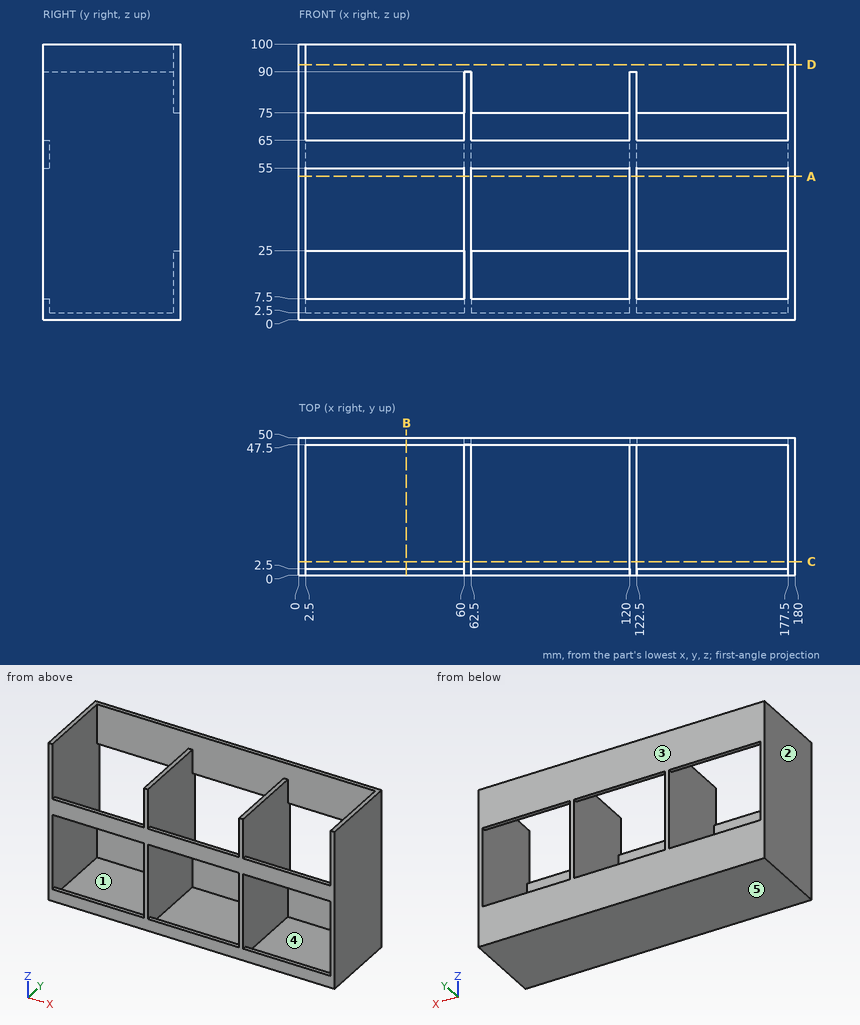
Could you check a few things on this drawing? It's one solid part, dimensions in mm from its lowest x, y, z. A direction names the side the tool comes from. Give positions to 0.01 mm unless a question says otherwise; leave off trailing zeros. Loops run counter-clockwise (first coordinate to the right, second up) from the corner with the lowest first, then second, coordinate; pieces in that order, holes last. Notation, with made-up numbers: M 33.5,10 L 48.5,10 A20 cw 48.5,35 Z; hole C 13,72.5 d9. An arc over 180 degrees is marked long. Answer as a JSON object with one key per item and string values.
Q1. Suppose I cut it at B-B, the plane x = 39. List the corners of the cut face in (y, z) for me.
Values found:
{"outline": "M 0,0 L 50,0 L 50,25 L 47.5,25 L 47.5,2.5 L 2.5,2.5 L 2.5,7.5 L 0,7.5 Z; M 0,55 L 2.5,55 L 2.5,65 L 0,65 Z; M 47.5,75 L 50,75 L 50,100 L 47.5,100 Z"}
Q2. Suppose I cut it at D-D, the plane z = 92.5. List the corners of the cut face in (x, y) for me.
Values found:
{"outline": "M 0,0 L 2.5,0 L 2.5,47.5 L 177.5,47.5 L 177.5,0 L 180,0 L 180,50 L 0,50 Z"}
Q3. For P1, Ø8, axis at y = 22.5, z = 55.5, coming from the -X side; P2, Ø22.5, axis at x = 96.5, y = 31.5, coming from the +Z side; P3, Ø3, axis at x = 85.5, y = 1.5, coming from the +Z side; P4, Ø11, axis at x = 82.5, z = 59.5, coming from the +Y side, each with a flat end and sliding along its axis, tell me the tip position at first contact or that it passes through.
Values found:
{"P1": "stops at x = 0", "P2": "stops at z = 2.5", "P3": "stops at z = 65", "P4": "stops at y = 2.5"}
Q4. If we mould it in two halves opening along X, with no side actions, what happens to the marked faces 1, 2 and 3? For each: pulls with the +X half, pulls with the -X half, needs draft (parallel to the pull), parting line crosses it, or undercut.
Values found:
{"face 1": "undercut", "face 2": "pulls with the -X half", "face 3": "needs draft"}
Q5. Suppose I cut it at A-A, the plane z = 52. List the corners of the cut face in (x, y) for me, plus the area to 3 significant figures.
Values found:
{"outline": "M 0,0 L 2.5,0 L 2.5,50 L 0,50 Z; M 60,0 L 62.5,0 L 62.5,50 L 60,50 Z; M 120,0 L 122.5,0 L 122.5,50 L 120,50 Z; M 177.5,0 L 180,0 L 180,50 L 177.5,50 Z", "area": "500 mm²"}
Q6. For the marked faces 4 and 5, which set-ups out of +Z, -Z, +X, -X, +Y, -Y let a thin tool reach every point of the face, with its end or its side?
Values found:
{"face 4": "+Z", "face 5": "-Z, +X, -X, +Y, -Y"}
Q7. If I drill on probe 1 along X at (y, z) = (11.5, 78.5); probe 2 along X at (y, z) = (5.5, 91); probe 3 along Z at (x, y) = (171, 41.5), over which ranges is the centre line in solid material (lowest first)? Write a range as [from, to].
Values found:
{"probe 1": "x = [0, 2.5], [60, 62.5], [120, 122.5], [177.5, 180]", "probe 2": "x = [0, 2.5], [177.5, 180]", "probe 3": "z = [0, 2.5]"}
Q8. Suppose I cut it at C-C, the plane y = 5. List the corners of the cut face in (x, z) for me, plus the area to 4 significant figures.
Values found:
{"outline": "M 0,0 L 180,0 L 180,100 L 177.5,100 L 177.5,2.5 L 122.5,2.5 L 122.5,90 L 120,90 L 120,2.5 L 62.5,2.5 L 62.5,90 L 60,90 L 60,2.5 L 2.5,2.5 L 2.5,100 L 0,100 Z", "area": "1,375 mm²"}
